from build123d import *

# Parameters (mm, degrees)
F1_DEPTH = 298.45
F2_W     = 1041.4
F2_H     = 1041.4
F3_DEPTH = 298.451


with BuildPart() as f1:
    # F0 (on Top) → F1 (new body)
    with BuildSketch(Plane.XY):
        with BuildLine():
            Line((-552.45, 476.25), (-546.1, 476.25))
            Line((-546.1, 476.25), (-546.1, -476.25))
            Line((-546.1, -476.25), (-552.45, -476.25))
            Line((-552.45, -476.25), (-552.45, -482.6))
            ThreePointArc((-552.45, -482.6), (-565.920384, -488.179616), (-571.5, -501.65))
            Line((-571.5, -501.65), (-577.85, -501.65))
            Line((-577.85, -501.65), (-577.85, -552.45))
            Line((-577.85, -552.45), (-571.5, -552.45))
            ThreePointArc((-571.5, -552.45), (-565.920384, -565.920384), (-552.45, -571.5))
            Line((-552.45, -571.5), (-552.45, -577.85))
            Line((-552.45, -577.85), (-501.65, -577.85))
            Line((-501.65, -577.85), (-501.65, -571.5))
            ThreePointArc((-501.65, -571.5), (-488.179616, -565.920384), (-482.6, -552.45))
            Line((-482.6, -552.45), (-476.25, -552.45))
            Line((-476.25, -552.45), (-476.25, -546.1))
            Line((-476.25, -546.1), (476.25, -546.1))
            Line((476.25, -546.1), (476.25, -552.45))
            Line((476.25, -552.45), (482.6, -552.45))
            ThreePointArc((482.6, -552.45), (488.179616, -565.920384), (501.65, -571.5))
            Line((501.65, -571.5), (501.65, -577.85))
            Line((501.65, -577.85), (552.45, -577.85))
            Line((552.45, -577.85), (552.45, -571.5))
            ThreePointArc((552.45, -571.5), (565.920384, -565.920384), (571.5, -552.45))
            Line((571.5, -552.45), (577.85, -552.45))
            Line((577.85, -552.45), (577.85, -501.65))
            Line((577.85, -501.65), (571.5, -501.65))
            ThreePointArc((571.5, -501.65), (565.920384, -488.179616), (552.45, -482.6))
            Line((552.45, -482.6), (552.45, -476.25))
            Line((552.45, -476.25), (546.1, -476.25))
            Line((546.1, -476.25), (546.1, 476.25))
            Line((546.1, 476.25), (552.45, 476.25))
            Line((552.45, 476.25), (552.45, 482.6))
            ThreePointArc((552.45, 482.6), (565.920384, 488.179616), (571.5, 501.65))
            Line((571.5, 501.65), (577.85, 501.65))
            Line((577.85, 501.65), (577.85, 552.45))
            Line((577.85, 552.45), (571.5, 552.45))
            ThreePointArc((571.5, 552.45), (565.920384, 565.920384), (552.45, 571.5))
            Line((552.45, 571.5), (552.45, 577.85))
            Line((552.45, 577.85), (501.65, 577.85))
            Line((501.65, 577.85), (501.65, 571.5))
            ThreePointArc((501.65, 571.5), (488.179616, 565.920384), (482.6, 552.45))
            Line((482.6, 552.45), (476.25, 552.45))
            Line((476.25, 552.45), (476.25, 546.1))
            Line((476.25, 546.1), (-476.25, 546.1))
            Line((-476.25, 546.1), (-476.25, 552.45))
            Line((-476.25, 552.45), (-482.6, 552.45))
            ThreePointArc((-482.6, 552.45), (-488.179616, 565.920384), (-501.65, 571.5))
            Line((-501.65, 571.5), (-501.65, 577.85))
            Line((-501.65, 577.85), (-552.45, 577.85))
            Line((-552.45, 577.85), (-552.45, 571.5))
            ThreePointArc((-552.45, 571.5), (-565.920384, 565.920384), (-571.5, 552.45))
            Line((-571.5, 552.45), (-577.85, 552.45))
            Line((-577.85, 552.45), (-577.85, 501.65))
            Line((-577.85, 501.65), (-571.5, 501.65))
            ThreePointArc((-571.5, 501.65), (-565.920384, 488.179616), (-552.45, 482.6))
            Line((-552.45, 482.6), (-552.45, 476.25))
        make_face()
    extrude(amount=F1_DEPTH)

    # F2 (on face) → F3 (cut, through all)
    with BuildSketch(Plane(origin=(0, 0, 0), x_dir=(1, 0, 0), z_dir=(0, 0, -1))):
        Rectangle(F2_W, F2_H)
    extrude(amount=-F3_DEPTH, mode=Mode.SUBTRACT)


solid = f1.part
Here's how the part is built. I have some questions about the finished solid (model axes, mm). A direction names the side the tool comes from. Give positions to 0.01 mm unless a question says otherwise; leave off trailing zeros. Loops run counter-clockwise (first coordinate to the right, second up) from the corner with the lowest first, then second, coordinate; pieces in that order, holes last. Notation, with made-up numbers: (-9.5, 24) -> (-3.5, 24) arc R26 ccw to (-3.5, 49) -> close; hole circle Ø8 at (6, 64). An arc over 180 degrees is marked (long way). Answer as a JSON object with one key per item and string values. Group by question number.
Item 1: On a 3-axis mill with a long thin cutter (end or side, diameter ignored), from which of +Z, -Z, +X, -X, +Y, -Y can I reach the whole of each face in a straight line? I mean faces 1 (the flat face through (-520.7, 7, 147)), 2 (the flat face through (-7, -546.1, 147)), 3 (the flat face through (546.1, -7, 147)), 4 (the flat face through (7, 546.1, 147)). Say none if no direction works.
Item 2: Imagine slicing it at A-A on y = 110. Write out the boundary of the cut face in (x, z).
Item 3: I need wall thicknesses on L1, parallel to X at y = 445, z = 178.5; L2, parallel to X at y = 513, z = 50.5. Which ranges of each line are inside material? Lowest first, please.
Item 4: Will these pins go through, and if not, where does the flat tip stop? pin 1 (1 mm diameter, centred on x = -344, z = 122, fed in from +Y); pin 2 (1.9 mm diameter, centred on x = 575.5, z = 83, fed in from -Y); pin 3 (5 mm diameter, centred on y = 454.5, z = 215.5, fed in from -X).
Item 5: Thinking about a two-plate mould opening in Y: for faces 5 (the flat face through (577.85, -527, 147)), 6 (the flat face through (-527, -577.85, 147)), 7 (the flat face through (-546.1, 7, 147)), which applies, pulls with the +Y half, pulls with the -Y half, needs draft (parallel to the pull), parting line crosses it, or undercut?
Answer list:
{
 "1": {"face 1": "+Z, -Z", "face 2": "+Z, -Z, -Y", "face 3": "+Z, -Z, +X", "face 4": "+Z, -Z, +Y"},
 "2": {"outline": "(-546.1, 0) -> (-520.7, 0) -> (-520.7, 298.45) -> (-546.1, 298.45) -> close; (520.7, 0) -> (546.1, 0) -> (546.1, 298.45) -> (520.7, 298.45) -> close"},
 "3": {"L1": "x = -546.1 to -520.7, 520.7 to 546.1", "L2": "x = -577.85 to -520.7, 520.7 to 577.85"},
 "4": {"pin 1": "stops at y = 546.1", "pin 2": "stops at y = -552.45", "pin 3": "stops at x = -546.1"},
 "5": {"face 5": "needs draft", "face 6": "pulls with the -Y half", "face 7": "undercut"}
}
